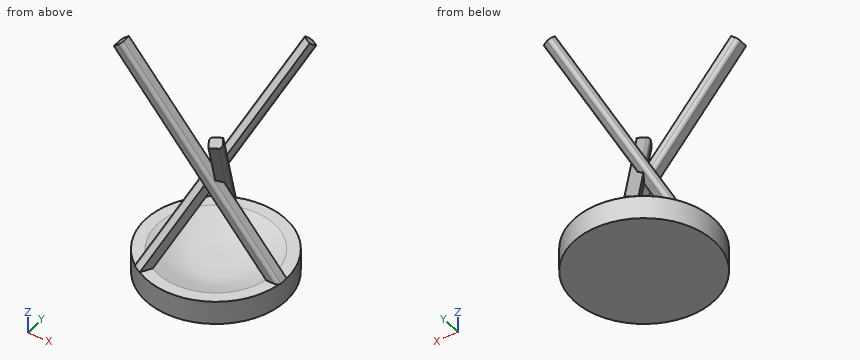
```python
from build123d import *

# Parameters (mm, degrees)
F0_W         = 5
F0_H         = 10
F3_DEPTH     = 5
F4_COUNT     = 3
F5_T4_DEPTH  = 64.961938704
F5_T9_DEPTH  = 108.2772549851
F5_T14_DEPTH = 111.6336535099
F5_T19_DEPTH = 111.6336535099
F5_T24_DEPTH = 64.3133444777
F5_T29_DEPTH = 64.3133444777
F5_T34_DEPTH = 108.2772549851


# Not quite as in the source:
# - a fillet or chamfer that OpenCascade refuses, or shapes differently, is made with other operations: its cross-section is extruded or revolved along the edge and cut away or added


with BuildPart() as f1:
    # F0 (on Front) → F1 (revolve)
    with BuildSketch(Plane.XZ):
        with Locations((-27.5, 5)):
            Rectangle(F0_W, F0_H)
        with BuildLine():
            Line((-25, 10), (-25, 0))
            Line((-25, 0), (0, 0))
            Line((0, 0), (0, 5))
            add(Edge.make_bspline(
                [(-25, 10), (-12.5, 5), (-12.5, 5), (0, 5)],
                knots=[0, 0, 0, 0, 25.495097568, 25.495097568, 25.495097568, 25.495097568], degree=3))
        make_face()
    revolve(axis=Axis((0, 0, 2.5), (0, 0, -1)))

    # F2 (on Front) → F3 (join)
    with BuildSketch(Plane.XZ):
        Polygon((24.7783708427, 10), (30, 10), (-36.9358222275, 89.7710066129), (-40, 87.1998561742), align=None)
    extrude(amount=F3_DEPTH)

    # F4: F1 ×3 about axis
    f4_axis = Axis((0, 0, 2.5), (0, 0, -1))


with BuildPart() as f1_1:
    add(f1.part)
    for i in range(1, F4_COUNT):
        add(f1.part.rotate(f4_axis, i * 360 / F4_COUNT))

    # F5: fillet of radius 1.5 on 7 edges, made by hand


with BuildPart() as f5_tool2:
    # F5_s3 → F5_t4 (new body)
    with BuildSketch(Plane(origin=(10.0591539469, -17.4229657171, 23.9760657093), x_dir=(0.8660254038, 0.5, 0), z_dir=(0.3213938048, -0.5566703992, 0.7660444431))):
        with BuildLine():
            ThreePointArc((1.5, 29.4092093904), (0.4393398282, 28.9698695622), (0, 27.9092093904))
            Line((0, 27.9092093904), (0, 29.4092093904))
            Line((0, 29.4092093904), (1.5, 29.4092093904))
        make_face()
    extrude(amount=F5_T4_DEPTH)

    split(bisect_by=Plane(origin=(22.5287614301, 0, 18.9038754068), x_dir=(0, 1, 0), z_dir=(0.7660444431, 0, 0.6427876097)), keep=Keep.TOP)


with BuildPart() as f1_2:
    add(f1_1.part)

    # F5_t1: cut F5_tool2
    add(f5_tool2.part, mode=Mode.SUBTRACT)


with BuildPart() as f5_tool7:
    # F5_s8 → F5_t9 (new body)
    with BuildSketch(Plane(origin=(30.937518597, -53.58535407, 73.7397978677), x_dir=(-0.8660254038, -0.5, 0), z_dir=(-0.3213938048, 0.5566703992, -0.7660444431))):
        with BuildLine():
            ThreePointArc((-5, 26.9092093904), (-4.5606601718, 25.8485492187), (-3.5, 25.4092093904))
            Line((-3.5, 25.4092093904), (-5, 25.4092093904))
            Line((-5, 25.4092093904), (-5, 26.9092093904))
        make_face()
    extrude(amount=F5_T9_DEPTH)

    split(bisect_by=Plane.XY.offset(10), keep=Keep.TOP)


with BuildPart() as f1_3:
    add(f1_2.part)

    # F5_t6: cut F5_tool7
    add(f5_tool7.part, mode=Mode.SUBTRACT)


with BuildPart() as f5_tool12:
    # F5_s13 → F5_t14 (new body)
    with BuildSketch(Plane(origin=(9.8816921063, 0, -11.7765420685), x_dir=(0, 1, 0), z_dir=(-0.6427876097, 0, 0.7660444431))):
        with BuildLine():
            ThreePointArc((-5, -27.9092093904), (-4.5606601718, -28.9698695622), (-3.5, -29.4092093904))
            Line((-3.5, -29.4092093904), (-5, -29.4092093904))
            Line((-5, -29.4092093904), (-5, -27.9092093904))
        make_face()
    extrude(amount=F5_T14_DEPTH)

    split(bisect_by=Plane.XY.offset(10), keep=Keep.TOP)


with BuildPart() as f1_4:
    add(f1_3.part)

    # F5_t11: cut F5_tool12
    add(f5_tool12.part, mode=Mode.SUBTRACT)


with BuildPart() as f5_tool17:
    # F5_s18 → F5_t19 (new body)
    with BuildSketch(Plane(origin=(-4.9408460531, -8.5577963964, -11.7765420685), x_dir=(-0.8660254038, 0.5, 0), z_dir=(0.3213938048, 0.5566703992, 0.7660444431))):
        with BuildLine():
            ThreePointArc((5, 27.9092093904), (4.5606601718, 28.9698695622), (3.5, 29.4092093904))
            Line((3.5, 29.4092093904), (5, 29.4092093904))
            Line((5, 29.4092093904), (5, 27.9092093904))
        make_face()
    extrude(amount=F5_T19_DEPTH)

    split(bisect_by=Plane.XY.offset(10), keep=Keep.TOP)


with BuildPart() as f1_5:
    add(f1_4.part)

    # F5_t16: cut F5_tool17
    add(f5_tool17.part, mode=Mode.SUBTRACT)


with BuildPart() as f5_tool22:
    # F5_s23 → F5_t24 (new body)
    with BuildSketch(Plane(origin=(-61.8750371939, 0, 73.7397978677), x_dir=(0, 1, 0), z_dir=(0.6427876097, 0, -0.7660444431))):
        with BuildLine():
            ThreePointArc((-1.5, 25.4092093904), (-0.4393398282, 25.8485492187), (0, 26.9092093904))
            Line((0, 26.9092093904), (0, 25.4092093904))
            Line((0, 25.4092093904), (-1.5, 25.4092093904))
        make_face()
    extrude(amount=F5_T24_DEPTH)

    split(bisect_by=Plane(origin=(-11.264380715, -19.5104797142, 18.9038754068), x_dir=(0.8660254038, -0.5, 0), z_dir=(-0.3830222216, -0.6634139482, 0.6427876097)), keep=Keep.TOP)


with BuildPart() as f1_6:
    add(f1_5.part)

    # F5_t21: cut F5_tool22
    add(f5_tool22.part, mode=Mode.SUBTRACT)


with BuildPart() as f5_tool27:
    # F5_s28 → F5_t29 (new body)
    with BuildSketch(Plane(origin=(30.937518597, 53.58535407, 73.7397978677), x_dir=(0.8660254038, -0.5, 0), z_dir=(-0.3213938048, -0.5566703992, -0.7660444431))):
        with BuildLine():
            ThreePointArc((0, 26.9092093904), (-0.4393398282, 25.8485492187), (-1.5, 25.4092093904))
            Line((-1.5, 25.4092093904), (0, 25.4092093904))
            Line((0, 25.4092093904), (0, 26.9092093904))
        make_face()
    extrude(amount=F5_T29_DEPTH)

    split(bisect_by=Plane(origin=(-11.264380715, 19.5104797142, 18.9038754068), x_dir=(-0.8660254038, -0.5, 0), z_dir=(-0.3830222216, 0.6634139482, 0.6427876097)), keep=Keep.TOP)


with BuildPart() as f1_7:
    add(f1_6.part)

    # F5_t26: cut F5_tool27
    add(f5_tool27.part, mode=Mode.SUBTRACT)


with BuildPart() as f5_tool32:
    # F5_s33 → F5_t34 (new body)
    with BuildSketch(Plane(origin=(30.937518597, 53.58535407, 73.7397978677), x_dir=(0.8660254038, -0.5, 0), z_dir=(-0.3213938048, -0.5566703992, -0.7660444431))):
        with BuildLine():
            ThreePointArc((-5, 26.9092093904), (-4.5606601718, 25.8485492187), (-3.5, 25.4092093904))
            Line((-3.5, 25.4092093904), (-5, 25.4092093904))
            Line((-5, 25.4092093904), (-5, 26.9092093904))
        make_face()
    extrude(amount=F5_T34_DEPTH)

    split(bisect_by=Plane.XY.offset(10), keep=Keep.TOP)


with BuildPart() as f1_8:
    add(f1_7.part)

    # F5_t31: cut F5_tool32
    add(f5_tool32.part, mode=Mode.SUBTRACT)


solid = f1_8.part
```
The listing builds one solid part. Answer for the finished solid, in the listing's coordinates (mm). Round coordinates to 2 decimals unless told otherwise and drop trailing zeros.
Q1. Given pin 1 Ø0.9 at (x, y) = (-13.5, -21) entering from -Z; pin 2 Ø9 at (x, y) = (-19.5, -2) entering from +Z; pin 3 Ø24 at (x, z) = (18, 33) entering from +Y; pin 4 Ø6 at (x, y) = (6.5, 10.5) entering from +Z, each flat-ended and moving along its own axis, determine where each tip first touches the part or whether it passes through.
Q2. Section A-A, the plane z = 23 is taken. Count the separate pieces of the cut face and the enclosed holes in it, then the cut area to 3 significant figures.
Q3. Find the intervals of material crossed by line 1 (Z direction, x = -3.5, y = -4); line 2 (Z direction, x = -27, y = 6); line 3 (Y direction, x = 13.5, z = 24), in increasing order.
Completed:
1. pin 1: stops at z = 0
1. pin 2: stops at z = 74.35
1. pin 3: stops at y = 0
1. pin 4: stops at z = 64.01
2. separate pieces: 3
2. enclosed holes: 0
2. area: 75.8 mm2
3. line 1: z = 0 to 5.02, 33.32 to 39.54, 43.7 to 49.79
3. line 2: z = 0 to 10
3. line 3: y = -5 to 0
